Study the drawing (mm; zero at the part's minimum x, y, z) and answer. Round coordinates to 2 decimals unless told otherwise and drop trailing zeros. Order: outer loops, then holes, each group sorted by start corner. A loop starts at its lowest first (then second) coordinate and runs counter-clockwise, first axis right, second up. Notation, with made-up numbers: (86, 80) - (104, 80) arc R25 ccw to (104, 101) - close; hole circle Ø10 at (35.25, 2.5). An arc over 180 degrees is marked (long way). Put each result on its own line as item: value. Start each with the question number.
Q1. Find the intervals of material crossed by line 1 along Z through (x, y) = (31, 22); line 2 along X through (y, z) = (8, 36.5); line 3 along X through (y, z) = (11, 31), in increasing order. Write a range as from..to.
Q2. For a pull along X with two mould halves and no side action, classify the marked faces 1, 2, 3 and 4 as pulls with the +X half, pulls with the -X half, needs draft (parallel to the pull), parting line crosses it, or undercut.
Q3. Section C-C on x = 19.5 is taken. Give the vertices of the cut face in (y, z).
Q4. Section D-D on z = 9 is taken. Give the vertices of the cut face in (x, y).
Q5. Each of these flat-tipped pins is pushed along its axis until it touches: pin 1 Ø5 at (x, y) = (14, 25) entering from -Z; pin 2 Ø1 at (y, z) = (12.5, 13) entering from -X; pin 3 Ø3 at (x, z) = (5, 5) entering from -Y. Where does it stop, or does it pass through?
Q6. Section A-A on y = 22 is taken. Give the vertices of the cut face in (x, z).
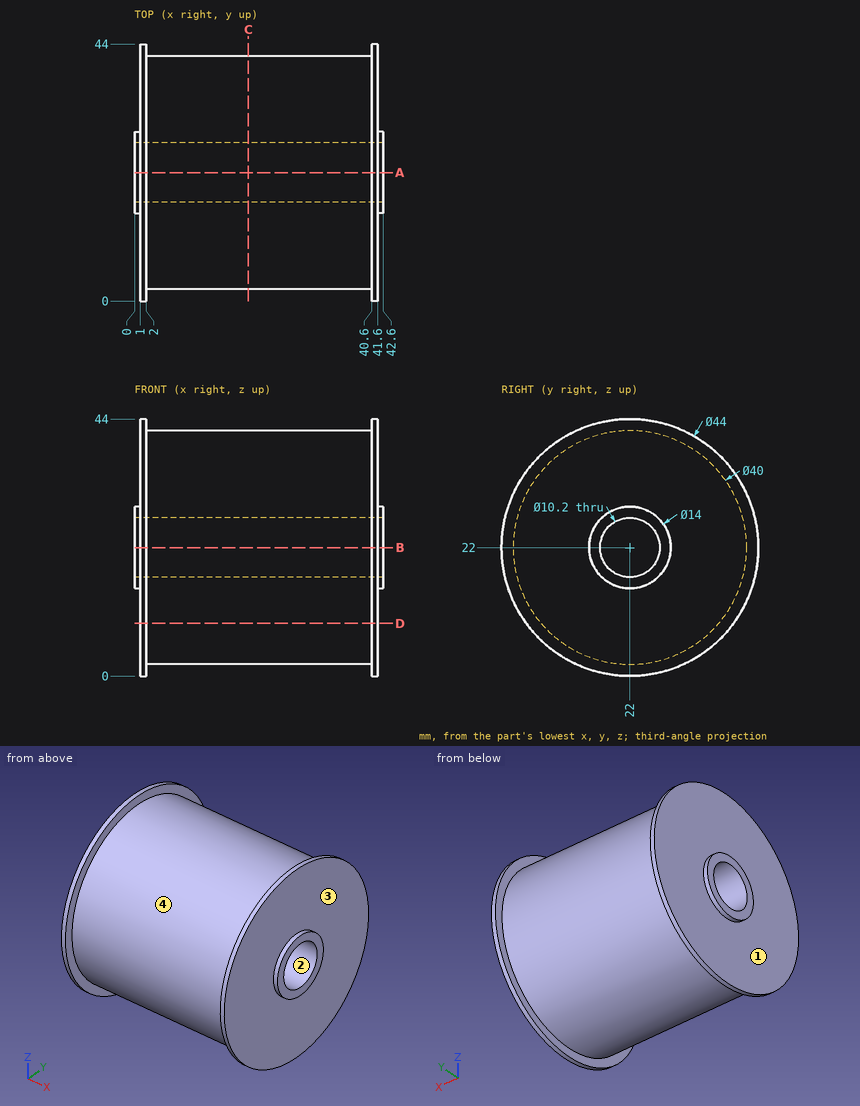
Findings:
1. line 1: 2..16.9, 27.1..42
1. line 2: 1..2, 40.6..41.6
1. line 3: 1..41.6
2. face 1: pulls with the -X half
2. face 2: needs draft
2. face 3: pulls with the +X half
2. face 4: undercut
3. outline: circle Ø40 at (22, 22); hole circle Ø10.2 at (22, 22)
4. outline: (1, 4.25) - (2, 4.25) - (2, 6.8) - (40.6, 6.8) - (40.6, 4.25) - (41.6, 4.25) - (41.6, 39.75) - (40.6, 39.75) - (40.6, 37.2) - (2, 37.2) - (2, 39.75) - (1, 39.75) - close
5. pin 1: z = 2.01
5. pin 2: x = 1
5. pin 3: y = 9.36
6. outline: (0, 15) - (1, 15) - (1, 0) - (2, 0) - (2, 2) - (40.6, 2) - (40.6, 0) - (41.6, 0) - (41.6, 15) - (42.6, 15) - (42.6, 16.9) - (0, 16.9) - close; (0, 27.1) - (42.6, 27.1) - (42.6, 29) - (41.6, 29) - (41.6, 44) - (40.6, 44) - (40.6, 42) - (2, 42) - (2, 44) - (1, 44) - (1, 29) - (0, 29) - close
